from build123d import *

# Parameters (mm, degrees)
F0_R     = 1.778
F0_R_2   = 1.524
F0_R_3   = 3.175
F1_DEPTH = 1.5875
F2_R     = 5.08


with BuildPart() as f1:
    # F0 (on Top) → F1 (new body)
    with BuildSketch(Plane.XY):
        with BuildLine():
            Line((-7.9375, -49.2125), (7.9375, -49.2125))
            Line((7.9375, -49.2125), (7.9375, 49.2125))
            ThreePointArc((7.9375, 49.2125), (0, 71.826434), (-7.9375, 49.2125))
            Line((-7.9375, 49.2125), (-7.9375, -49.2125))
        make_face()
        with Locations((0, -42.8625)):
            Circle(F0_R, mode=Mode.SUBTRACT)
        with Locations((0, -31.75)):
            Circle(F0_R, mode=Mode.SUBTRACT)
        with Locations((-9.5, 59.126434)):
            Circle(F0_R_2, mode=Mode.SUBTRACT)
        with Locations((-4.75, 50.899193)):
            Circle(F0_R_2, mode=Mode.SUBTRACT)
        with Locations((-4.75, 67.353676)):
            Circle(F0_R_2, mode=Mode.SUBTRACT)
        with Locations((0, 39.6875)):
            Circle(F0_R_3, mode=Mode.SUBTRACT)
        with Locations((4.75, 50.899193)):
            Circle(F0_R_2, mode=Mode.SUBTRACT)
        with Locations((4.75, 67.353676)):
            Circle(F0_R_2, mode=Mode.SUBTRACT)
        with Locations((9.5, 59.126434)):
            Circle(F0_R_2, mode=Mode.SUBTRACT)
    extrude(amount=F1_DEPTH)

    # F2
    f2_edges = [f1.edges().sort_by_distance(p)[0] for p in [
        (7.9375, 49.2125, 0.79375),
        (7.9375, -49.2125, 0.79375),
        (-7.9375, -49.2125, 0.79375),
        (-7.9375, 49.2125, 0.79375),
    ]]
    fillet(f2_edges, radius=F2_R)


solid = f1.part
CAD build for the part. Positions are in the model's coordinates, mm. Give positions to 0.01 mm unless a question says otherwise; leave off trailing zeros. Loops run counter-clockwise (first coordinate to the right, second up) from the corner with the lowest first, then second, coordinate; pieces in that order, holes last. Notation, with made-up numbers: M -38.5,26 L -28.5,26 A20 ccw -28.5,57 Z; hole C 47,33 d9. An arc over 180 degrees is marked long. Answer in a Markdown table with one row per item. Add a question column.
Item 1: Mould opens along Y. For faces 1 (the face through (10.32, 60.41, 0.78)), 2 (the face through (0, 12, 1.588)), 3 (the face through (6.41, -47.764, 0.805)) say: +Y half, -Y half, draft (parallel to the pull), parting line (faces both ways), or undercut.
Item 2: Band-saw the part on C-C on x = 0. Give the cut face in (y, z), then the cut area to 3 significant figures.
Item 3: Band-saw the part on D-D on z = 0.75. Give the number of separate pieces and of enclosed holes in the cut face, then the cut area to 3 significant figures.
Item 4: Band-saw the part on B-B on x = -4.75. Give the cut face in (y, z).
Item 5: Drop a flat-ended pin along its axis: P1, Ø0.8, axis at y = -7.5, z = 1, coming from the -X side. Give the stop position or say it passes through.
Item 6: Band-saw the part on A-A on y = -31.75. Give the cut face in (x, z).
Item 7: Probe probe 1 along Y at (x, z) = (0, 1); probe 2 along X at (y, z) = (50, 0.8); probe 3 along X at (y, z) = (60, 0.95). List the from-to ranges inside material, lowest first.
Reply:
| question | item | result |
|---|---|---|
| 1 | face 1 | undercut |
| 1 | face 2 | draft |
| 1 | face 3 | -Y half |
| 2 | outline | M -49.21,0 L -44.64,0 L -44.64,1.59 L -49.21,1.59 Z; M -41.08,0 L -33.53,0 L -33.53,1.59 L -41.08,1.59 Z; M -29.97,0 L 36.51,0 L 36.51,1.59 L -29.97,1.59 Z; M 42.86,0 L 71.83,0 L 71.83,1.59 L 42.86,1.59 Z |
| 2 | area | 171 mm^2 |
| 3 | separate pieces | 1 |
| 3 | enclosed holes | 9 |
| 3 | area | 1,930 mm^2 |
| 4 | outline | M -48.85,0 L 49.38,0 L 49.38,1.59 L -48.85,1.59 Z; M 52.42,0 L 65.83,0 L 65.83,1.59 L 52.42,1.59 Z; M 68.88,0 L 70.9,0 L 70.9,1.59 L 68.88,1.59 Z |
| 5 | P1 | stops at x = -7.94 |
| 6 | outline | M -7.94,0 L -1.78,0 L -1.78,1.59 L -7.94,1.59 Z; M 1.78,0 L 7.94,0 L 7.94,1.59 L 1.78,1.59 Z |
| 7 | probe 1 | y = -49.21 to -44.64, -41.08 to -33.53, -29.97 to 36.51, 42.86 to 71.83 |
| 7 | probe 2 | x = -8.91 to -5.98, -3.52 to 3.52, 5.98 to 8.91 |
| 7 | probe 3 | x = -12.67 to -10.75, -8.25 to 8.25, 10.75 to 12.67 |
